```python
from build123d import *

# Parameters (mm, degrees)
F0_R     = 11.25
F1_DEPTH = 7
F2_R     = 3


with BuildPart() as f1:
    # F0 (on Front) → F1 (new body)
    with BuildSketch(Plane.XZ):
        with BuildLine():
            ThreePointArc((5.8359223436, -14.0891628708), (12.6799115876, -8.4724460535), (15.25, 0))
            ThreePointArc((15.25, 0), (12.6799115876, 8.4724460535), (5.8359223436, 14.0891628708))
            ThreePointArc((5.8359223436, 14.0891628708), (0, 15.25), (-5.8359223436, 14.0891628708))
            ThreePointArc((-5.8359223436, 14.0891628708), (-12.6799115876, 8.4724460535), (-15.25, 0))
            ThreePointArc((-15.25, 0), (-12.6799115876, -8.4724460535), (-5.8359223436, -14.0891628708))
            ThreePointArc((-5.8359223436, -14.0891628708), (0, -15.25), (5.8359223436, -14.0891628708))
        make_face()
        Circle(F0_R, mode=Mode.SUBTRACT)
        with BuildLine():
            Line((15.25, -25), (15.25, 0))
            ThreePointArc((15.25, 0), (12.6799115876, -8.4724460535), (5.8359223436, -14.0891628708))
            Line((5.8359223436, -14.0891628708), (15.25, -25))
        make_face()
        with BuildLine():
            ThreePointArc((5.8359223436, 14.0891628708), (12.6799115876, 8.4724460535), (15.25, 0))
            Line((15.25, 0), (15.25, 25))
            Line((15.25, 25), (5.8359223436, 14.0891628708))
        make_face()
        Polygon((15.25, 25), (15.25, 0), (15.25, -25), (65.25, 0), align=None)
        with Locations((33.02, 0)):
            Circle(F0_R, mode=Mode.SUBTRACT)
        with BuildLine():
            ThreePointArc((-15.25, 0), (-12.6799115876, 8.4724460535), (-5.8359223436, 14.0891628708))
            Line((-5.8359223436, 14.0891628708), (-15.25, 25))
            Line((-15.25, 25), (-15.25, 0))
        make_face()
        with BuildLine():
            Line((-15.25, -25), (-5.8359223436, -14.0891628708))
            ThreePointArc((-5.8359223436, -14.0891628708), (-12.6799115876, -8.4724460535), (-15.25, 0))
            Line((-15.25, 0), (-15.25, -25))
        make_face()
        Polygon((-15.25, -25), (-15.25, 0), (-15.25, 25), (-65.25, 0), align=None)
        with Locations((-33.02, 0)):
            Circle(F0_R, mode=Mode.SUBTRACT)
    extrude(amount=F1_DEPTH)

    # F2
    f2_edges = [f1.edges().sort_by_distance(p)[0] for p in [
        (-15.25, -3.5, -25),
        (-5.835922, -3.5, -14.089163),
        (-10.542961, 0, -19.544581),
        (-10.542961, -7, -19.544581),
        (5.835922, -3.5, -14.089163),
        (0, 0, -15.25),
        (0, -7, -15.25),
        (15.25, -3.5, -25),
        (10.542961, 0, -19.544581),
        (10.542961, -7, -19.544581),
        (-65.25, -3.5, 0),
        (-40.25, 0, -12.5),
        (-40.25, -7, -12.5),
        (65.25, -3.5, 0),
        (40.25, 0, -12.5),
        (40.25, -7, -12.5),
        (15.25, -3.5, 25),
        (40.25, 0, 12.5),
        (40.25, -7, 12.5),
        (5.835922, -3.5, 14.089163),
        (10.542961, 0, 19.544581),
        (10.542961, -7, 19.544581),
        (-5.835922, -3.5, 14.089163),
        (0, 0, 15.25),
        (0, -7, 15.25),
        (-15.25, -3.5, 25),
        (-10.542961, 0, 19.544581),
        (-10.542961, -7, 19.544581),
        (-40.25, 0, 12.5),
        (-40.25, -7, 12.5),
    ]]
    fillet(f2_edges, radius=F2_R)


solid = f1.part
```
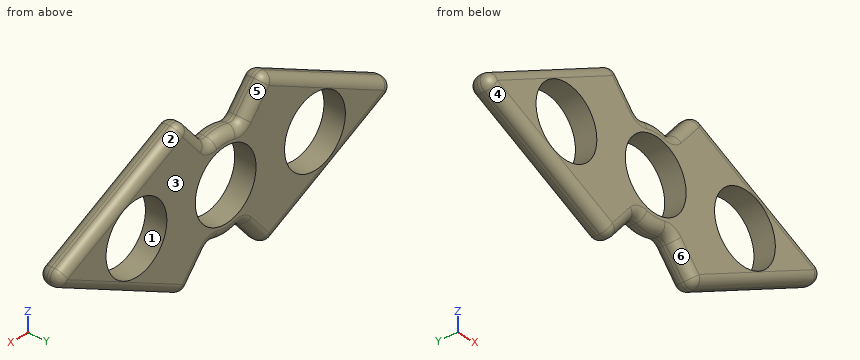
For this review, take the finished solid that the model builds, in its own axes (mm). Face numbers are marked on the shaded views. A direction names the side the tool comes from. Round coordinates to 2 decimals unless told otherwise and drop trailing zeros. Write each loop counter-clockwise with the first axis right and the second up, starting at its lowest first coordinate (ties: lowest second). Pieces come first, ordered by that corner, then holes. Notation, with made-up numbers: (-14.75, -0.5) - (-4.75, -0.5) arc R12 cw to (-4.75, 3.5) - close; hole circle Ø8 at (14.5, 3.5). An arc over 180 degrees is marked (long way). Write each question's results on one line, items separated by ' | '.
Item 1: Draft analysis for pull direction Z (two halves, no side actions). For the marked faces 1, 2 and 3, state which applies: pulls with the +Z half, pulls with the -Z half, needs draft (parallel to the pull), parting line crosses it, or undercut.
Calculated:
face 1: undercut | face 2: pulls with the +Z half | face 3: needs draft
Item 2: Take a section at A-A on x = 0. State the section outline as (y, z) points, then the cut area to 3 significant figures.
Calculated:
outline: (-7, -12.25) arc R3 ccw to (-4, -15.25) - (-3, -15.25) arc R3 ccw to (0, -12.25) - (0, -11.25) - (-7, -11.25) - close; (-7, 11.25) - (0, 11.25) - (0, 12.25) arc R3 ccw to (-3, 15.25) - (-4, 15.25) arc R3 ccw to (-7, 12.25) - close | area: 48.3 mm^2
Item 3: Take a section at B-B on y = -1.5. State the section outline as (x, z) points, then the cut area to 3 significant figures.
Calculated:
outline: (-59.7, -2.32) - (-17.16, -23.6) arc R2.6 ccw to (-14.03, -22.97) - (-7.46, -15.36) arc R3.4 cw to (-3.98, -14.31) arc R14.85 ccw to (3.98, -14.31) arc R3.4 cw to (7.46, -15.36) - (14.03, -22.97) arc R2.6 ccw to (17.16, -23.6) - (59.7, -2.32) arc R2.6 ccw to (59.7, 2.32) - (17.16, 23.6) arc R2.6 ccw to (14.03, 22.97) - (7.46, 15.36) arc R3.4 cw to (3.98, 14.31) arc R14.85 ccw to (-3.98, 14.31) arc R3.4 cw to (-7.46, 15.36) - (-14.03, 22.97) arc R2.6 ccw to (-17.16, 23.6) - (-59.7, 2.32) arc R2.6 ccw to start; hole circle Ø22.5 at (-33.02, 0); hole circle Ø22.5 at (0, 0); hole circle Ø22.5 at (33.02, 0) | area: 2,260 mm^2
Item 4: For the marked faces 4, 5 and 6, list the 3-axis set-ups (+Z, -Z, +X, -X, +Y, -Y) from which the entire face can be reached by the end or side of a thin tool; tool diameter is ignored.
Calculated:
face 4: -Z, -X, -Y | face 5: +Z, +Y | face 6: -Z, -Y
Item 5: For pin 1 (3 mm diameter, centred on y = -2.5, z = -8, fed in from +X); pin 2 (13.5 mm diameter, centred on x = 0, z = 0, fed in from +Y); pin 3 (3 mm diameter, centred on y = -5, z = -15.5, fed in from -X); pin 4 (4 mm diameter, centred on y = -1, z = 8, fed in from +X), all flat-tipped, find the tip position at first contact; note any pin that passes through.
Calculated:
pin 1: stops at x = 52.19 | pin 2: passes through | pin 3: stops at x = -37.01 | pin 4: stops at x = 52.36
Item 6: To check wall thickness, follow line 1 along Z through (x, y) = (0, -3.5); line 2 along X through (y, z) = (-4.5, -1.5); line 3 along X through (y, z) = (-4.5, -10). State the ranges of each line that lie inside material, in increasing order. Write a range as from..to.
Calculated:
line 1: z = -15.25..-11.25, 11.25..15.25 | line 2: x = -61.09..-44.17, -21.87..-11.15, 11.15..21.87, 44.17..61.09 | line 3: x = -45.16..-38.17, -27.87..-5.15, 5.15..27.87, 38.17..45.16
